Can you work these out from the drawing? Everything is in mm from the part's minimum corner. A direction names the side the tool comes from. Round coordinates to 2 decimals unless told otherwise and drop trailing zeros. Order: outer loops, then holes, each group sorted by start corner. A loop starts at its lowest first (then second) coordinate and runs counter-clockwise, first axis right, second up. Notation, with made-up numbers: M 25.25,-19 L 66.25,-19 A9 cw 66.25,-4 Z; hole C 8,-15 d5. An arc over 180 degrees is marked long. Write each question's results on one line, items separated by ' | '. Start each with the question number.
1. Suppose I cut it at D-D on y = 64. Write out the boundary of the cut face in (x, z), and give its area (3 significant figures).
2. Suppose I cut it at B-B on z = 31. Write out the boundary of the cut face in (x, y).
3. Suppose I cut it at C-C on y = 44.5. Write out the boundary of the cut face in (x, z), and give its area (3 significant figures).
4. For the marked faces 1, 2 and 3, which set-ups out of +Z, -Z, +X, -X, +Y, -Y let a thin tool reach every point of the face, with its end or its side?
5. Please list where these lines run through material, in increasing order: L1, parallel to X at y = 54, z = 13; L2, parallel to Z at x = 99.5, y = 43; L3, parallel to Z at x = 126, y = 64.
6. We'd pull the mould along X, two halves only. Please class the marked faces 4, 5 and 6: released by +X, released by -X, zero draft, split by the parting line, or undercut.
7. Suppose I cut it at A-A on x = 103.5. Write out the boundary of the cut face in (y, z).
8. I'm going to push flat-ended pins straight in: pin 1 (10 mm diameter, centred on y = 20.5, z = 78, fed in from +X); pin 2 (16 mm diameter, centred on x = 12.5, y = 20.5, fed in from -Z); pin 3 (1.5 mm diameter, centred on x = 180.5, y = 75.5, fed in from +Z). Where does each tip first touch, or does it pass through?
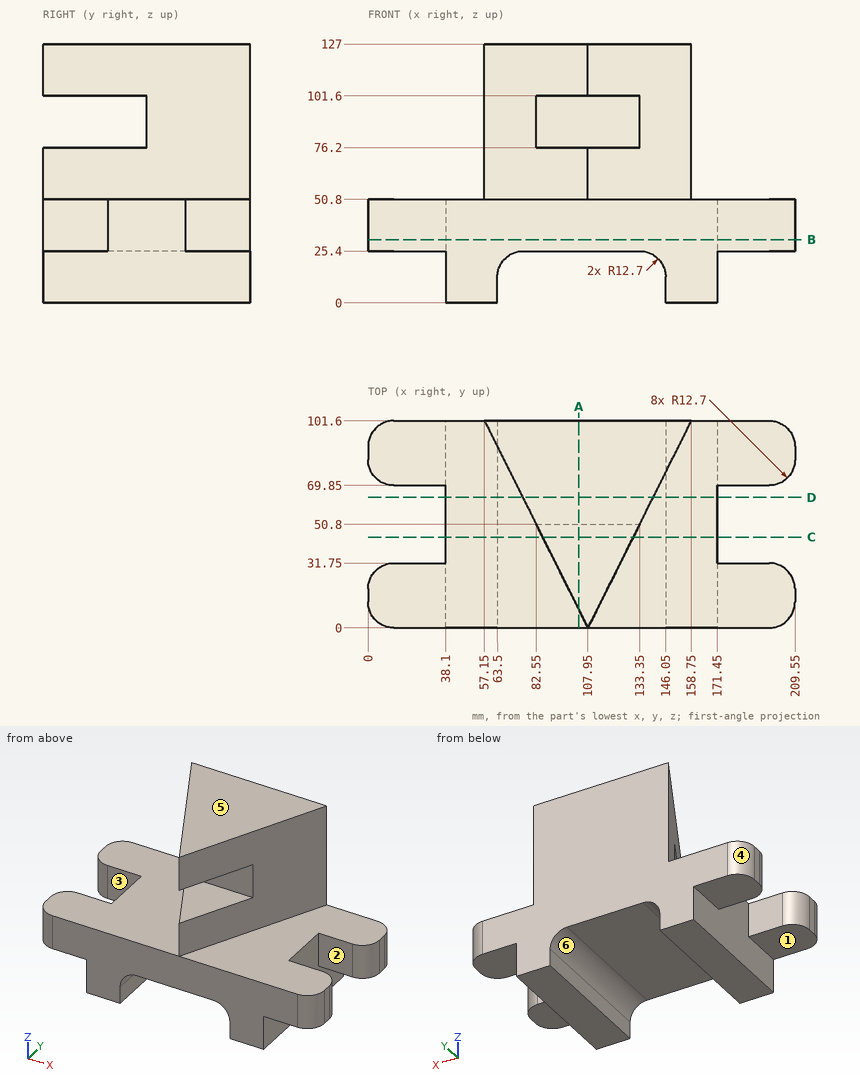
Filled sheet:
1) outline: M 38.1,0 L 63.5,0 L 63.5,12.7 A12.7 cw 76.2,25.4 L 133.35,25.4 A12.7 cw 146.05,12.7 L 146.05,0 L 171.45,0 L 171.45,50.8 L 139.95,50.8 L 139.95,127 L 75.95,127 L 75.95,50.8 L 38.1,50.8 Z | area: 9,620 mm^2
2) outline: M 0,12.7 A12.7 ccw 12.7,0 L 196.85,0 A12.7 ccw 209.55,12.7 L 209.55,19.05 A12.7 ccw 196.85,31.75 L 171.45,31.75 L 171.45,69.85 L 196.85,69.85 A12.7 ccw 209.55,82.55 L 209.55,88.9 A12.7 ccw 196.85,101.6 L 12.7,101.6 A12.7 ccw 0,88.9 L 0,82.55 A12.7 ccw 12.7,69.85 L 38.1,69.85 L 38.1,31.75 L 12.7,31.75 A12.7 ccw 0,19.05 Z
3) outline: M 38.1,0 L 63.5,0 L 63.5,12.7 A12.7 cw 76.2,25.4 L 133.35,25.4 A12.7 cw 146.05,12.7 L 146.05,0 L 171.45,0 L 171.45,50.8 L 130.2,50.8 L 130.2,76.2 L 85.7,76.2 L 85.7,50.8 L 38.1,50.8 Z; M 85.7,101.6 L 130.2,101.6 L 130.2,127 L 85.7,127 Z | area: 7,010 mm^2
4) face 1: -Z, -X, +Y, -Y | face 2: +Z, -Z, +X | face 3: +Z, -Z, -X
5) L1: x = 38.1 to 63.5, 146.05 to 171.45 | L2: z = 25.4 to 76.2, 101.6 to 127 | L3: z = 25.4 to 127
6) face 4: released by -X | face 5: zero draft | face 6: undercut
7) outline: M 0,25.4 L 101.6,25.4 L 101.6,127 L 8.9,127 L 8.9,101.6 L 50.8,101.6 L 50.8,76.2 L 8.9,76.2 L 8.9,50.8 L 0,50.8 Z
8) pin 1: stops at x = 120.53 | pin 2: stops at z = 25.4 | pin 3: stops at z = 50.8
